CAD build for the part. Positions are in the model's coordinates, mm. A direction names the side the tool comes from. Round coordinates to 2 decimals unless told otherwise and drop trailing zeros. Order: outer loops, then holes, each group sorted by start corner. A loop starts at its lowest first (then second) coordinate and runs counter-clockwise, first axis right, second up.
```python
from build123d import *

# Parameters (mm, degrees)
SKETCH1_W           = 78
SKETCH1_H           = 34
BOSS_EXTRUDE1_DEPTH = 7
BOSS_EXTRUDE2_DEPTH = 7
BOSS_EXTRUDE3_DEPTH = 7
SKETCH6_W           = 70
SKETCH6_H           = 38
BOSS_EXTRUDE4_DEPTH = 7
CUT_EXTRUDE1_DEPTH  = 7


with BuildPart() as part:
    # Sketch1 → Boss-Extrude1 (new body)
    with BuildSketch(Plane(origin=(0, 0, 0), x_dir=(1, 0, 0), z_dir=(0, 1, 0))):
        Rectangle(SKETCH1_W, SKETCH1_H)
    extrude(amount=BOSS_EXTRUDE1_DEPTH)

    # Sketch3 → Boss-Extrude2 (add)
    with BuildSketch(Plane.ZY.offset(39)):
        Polygon((17, 7), (-17, 37.819553073), (-17, 7), align=None)
    extrude(amount=-BOSS_EXTRUDE2_DEPTH)

    # Sketch4 → Boss-Extrude3 (add)
    with BuildSketch(Plane(origin=(0, 0, -17), x_dir=(-1, 0, 0), z_dir=(0, 0, -1))):
        Polygon((-39, 0), (-39, 33), (39, 69.371997336), (39, 0), align=None)
    extrude(amount=BOSS_EXTRUDE3_DEPTH)

    # Sketch6 → Boss-Extrude4 (add)
    with BuildSketch(Plane(origin=(19.605374923, 42.043862201, 0), x_dir=(0.9063077870366493, -0.4226182617407009, 0), z_dir=(0.4226182617407009, 0.9063077870366493, 0))):
        with Locations((-21.632137783, 43)):
            Rectangle(SKETCH6_W, SKETCH6_H)
    extrude(amount=-BOSS_EXTRUDE4_DEPTH)

    # Sketch7 → Cut-Extrude1 (cut)
    with BuildSketch(Plane(origin=(19.605374923, 42.043862201, 0), x_dir=(0.9063077870366493, -0.4226182617407009, 0), z_dir=(0.4226182617407009, 0.9063077870366493, 0))):
        with BuildLine():
            Line((-14.694395531, 38), (-36.632137783, 38))
            ThreePointArc((-36.632137783, 38), (-40.632137783, 42), (-36.632137783, 46))
            Line((-36.632137783, 46), (-14.694395531, 46))
            ThreePointArc((-14.694395531, 46), (2.367862217, 42), (-14.694395531, 38))
        make_face()
    extrude(amount=-CUT_EXTRUDE1_DEPTH, mode=Mode.SUBTRACT)


solid = part.part
```
1. Cut at C-C, the plane x = -24. Write the cut outline in (y, z), and give its area (3 significant figures).
2. Tool access for faces 1 (the face through (30.262, 33.267, -42.734)), 2 (the face through (-33.18, 62.85, -42.73)), 3 (the face through (-32, 16, -8)), 4 (the face through (-3.4, 45.05, -47.49)): list every direction of +Z, -Z, +X, -X, +Y, -Y with a clear straight run to the whole face (end or side of a thin tool).
3. Cut at A-A, the plane x = -11.5. Write the cut outline in (y, z), and give its area (3 significant figures).
4. Cut at B-B, the plane z = -49.5. Write the cut outline in (x, y), and give its area (3 significant figures).
5. Mould opens along Z. For faces 5 (the face through (-5, 50, -38)), 6 (the face through (-35.55, 22.19, 0.24)), 7 (the face through (-1, 0, -3)) say: released by +Z, released by -Z, zero draft, split by the parting line, or undercut.
6. Drill centre lines: line 1 (Z direction, x = -10.5, y = 55); line 2 (Z direction, x = 30, y = 8.5); line 3 (Z direction, x = -32, y = 62.5). Where is each one in solid material? Low to high.
7. Cut at D-D, the plane y = 28.5. Write the cut outline in (x, z).
8. Pin check, flat tips, straight feed: P1, Ø2, axis at y = 17, z = -4.5, coming from the +X side; P2, Ø4, axis at x = -9.5, y = 41.5, coming from the +Z side. Stop position of each tip, or through.
Outcome:
1. outline: (0, -24) - (54.65, -24) - (54.65, -62) - (62.38, -62) - (62.38, -17) - (7, -17) - (7, 17) - (0, 17) - close
1. area: 968 mm2
2. face 1: -Z, +X, -Y
2. face 2: -Z, -X, +Y
2. face 3: +Z, +X, +Y
2. face 4: -Z, -X, -Y
3. outline: (0, -24) - (48.82, -24) - (48.82, -38) - (56.55, -38) - (56.55, -17) - (7, -17) - (7, 17) - (0, 17) - close; (48.82, -62) - (56.55, -62) - (56.55, -46) - (48.82, -46) - close
3. area: 866 mm2
4. outline: (-34.68, 59.63) - (6.13, 40.61) - (9.09, 46.95) - (-31.72, 65.98) - close; (15.15, 36.4) - (28.76, 30.05) - (31.72, 36.39) - (18.1, 42.74) - close
4. area: 420 mm2
5. face 5: undercut
5. face 6: released by +Z
5. face 7: zero draft
6. line 1: z = -62 to -46, -38 to -17
6. line 2: z = -24 to -17
6. line 3: z = -62 to -17
7. outline: (-39, -24) - (39, -24) - (39, -17) - (-32, -17) - (-32, -6.72) - (-39, -6.72) - close
8. P1: stops at x = -32
8. P2: stops at z = -17
